Read the model definition and answer for the solid it produces. Units are mm, in the model's axes. A direction names the side the tool comes from. Give positions to 0.01 mm unless a question says otherwise; leave off trailing zeros. Loops run counter-clockwise (first coordinate to the right, second up) from the corner with the lowest first, then second, coordinate; pieces in that order, holes last. Notation, with made-up numbers: (36.5, 14) -> (49.5, 14) arc R7 cw to (49.5, 27) -> close; hole circle Ø5 at (59, 18). An arc over 180 degrees is marked (long way). Write each question's results on one line, items separated by ' | '. Start each with the question number.
Item 1: Which of the six approach directions +Z, -Z, +X, -X, +Y, -Y give full straight-line access (tool end or side, diameter ignored) to faces 1 (the flat face through (18.374, 8.986, 14.113)), 2 (the cylindrical face through (17.1, 1.97, 14.43)), 3 (the cylindrical face through (17.1, 2.29, 3.98)), 4 (the flat face through (22, 9, 1.5))?
Item 2: Each of these flat-tipped pins is pushed along its axis until it touches: P1, Ø2.5, axis at x = 16.65, y = 10, coming from the +Z side; P2, Ø2, axis at x = 24, y = 9.5, coming from the -Z side; P3, Ø1, axis at y = 3, z = 2.5, coming from the -X side. Where does it stop, or does it pass through?
Item 3: Section C-C on x = -4 is taken. Write down the section's boundary in (y, z), and give its area (3 significant figures).
Item 4: Find the intervals of material crossed by line 1 (X direction, y = 7.5, z = 7.5); line 2 (X direction, y = 1.3, z = 7.5); line 3 (X direction, y = 6.75, z = 11.5), in increasing order.
Item 5: Section A-A on x = 32.7 is taken. Write down the section's boundary in (y, z) (3 decimals).
Item 6: Section B-B on x = 17 is taken. State how many separate pieces and enclosed holes the cut face has, and give its area (3 significant figures).
Item 7: Determine the mould class of faces 5 (the flat face through (4, 4, 8)), 6 (the flat face through (23, 12, 14)), 7 (the cylindrical face through (46.727, 2.535, 7.142)) for opening direction Y: +Y half, -Y half, draft (parallel to the pull), parting line (faces both ways), or undercut.
```python
from build123d import *

# Parameters (mm, degrees)
SKETCH1_W                = 40
SKETCH1_H                = 13
SWITCHCASE_DEPTH         = 15
SKETCH2_W                = 13
SKETCH2_H                = 5.9
SWITCHCAVITY_DEPTH       = 45.654227124
SWITCHM2HOLES_DEPTH      = 44.338233697
SWITCHM2HOLES_DEPTH_BACK = 44.338233697
SKETCH3_R                = 1.05
SKETCH14_R               = 2
M2HEAD_DEPTH             = 1.5
M2NUTINSERTS_DEPTH       = 45.654227124
M2NUTINSERTS_DEPTH_BACK  = 1.75
SKETCH7_W                = 15
SKETCH7_H                = 13
WINGS_DEPTH              = 15
M5NUTS_DEPTH             = 4
SKETCH10_R               = 3.05
M6HOLE_DEPTH             = 59.472215624
WIRECHANNEL_DEPTH        = 58.473493891
WIRECHANNEL_DEPTH_BACK   = 58.473493891
SKETCH11_W               = 4.6
SKETCH11_H               = 4
CHANNELFILLET_R          = 2
M5HEAD_DEPTH             = 59.472215624
M5HEAD_DEPTH_BACK        = 8
SKETCH12_R               = 4.5
SKETCH13_R               = 2.75
M5THREAD_DEPTH           = 59.472215624
ENDFILLET_R              = 5


with BuildPart() as part:
    # Sketch1 → SwitchCase (new body)
    with BuildSketch(Plane.XY):
        with Locations((20, 6.5)):
            Rectangle(SKETCH1_W, SKETCH1_H)
    extrude(amount=SWITCHCASE_DEPTH)

    # Sketch2 → SwitchCavity (cut, through all)
    with BuildSketch(Plane(origin=(0, 13, 0), x_dir=(1, 0, 0), z_dir=(0, 1, 0))):
        with Locations((20, -7.5)):
            Rectangle(SKETCH2_W, SKETCH2_H)
    extrude(amount=-SWITCHCAVITY_DEPTH, mode=Mode.SUBTRACT)

    # Sketch3 → SwitchM2Holes (cut, two sides: drawn at the far end of the back side and taken through both)
    with BuildSketch(Plane.XY.offset(4.55).offset(-SWITCHM2HOLES_DEPTH_BACK)):
        with Locations((16.65, 10)):
            Circle(SKETCH3_R)
        with Locations((23.35, 10)):
            Circle(SKETCH3_R)
    extrude(amount=SWITCHM2HOLES_DEPTH + SWITCHM2HOLES_DEPTH_BACK, mode=Mode.SUBTRACT)

    # Sketch14 → M2Head (cut)
    with BuildSketch(Plane(origin=(0, 0, 0), x_dir=(-1, 0, 0), z_dir=(0, 0, -1))):
        with Locations((-23.35, 10)):
            Circle(SKETCH14_R)
        with Locations(Location((-16.65, 10, 0), (0, 0, 180))):
            Circle(SKETCH14_R)
    extrude(amount=-M2HEAD_DEPTH, mode=Mode.SUBTRACT)

    # Sketch5 → M2NutInserts (cut, two sides: drawn at the far end of the back side and taken through both)
    with BuildSketch(Plane.XY.offset(15).offset(-M2NUTINSERTS_DEPTH_BACK)):
        Polygon((18.959401077, 10), (17.804700538, 12), (15.495299462, 12), (14.340598923, 10), (15.495299462, 8), (17.804700538, 8), align=None)
        Polygon((25.659401077, 10), (24.504700538, 12), (22.195299462, 12), (21.040598923, 10), (22.195299462, 8), (24.504700538, 8), align=None)
    extrude(amount=M2NUTINSERTS_DEPTH + M2NUTINSERTS_DEPTH_BACK, mode=Mode.SUBTRACT)

    # Sketch7 → Wings (add)
    with BuildSketch(Plane.XY.offset(15)):
        with Locations((-7.5, 6.5)):
            Rectangle(SKETCH7_W, SKETCH7_H)
        with Locations((47.5, 6.5)):
            Rectangle(SKETCH7_W, SKETCH7_H)
    extrude(amount=-WINGS_DEPTH)

    # Sketch9 → M5Nuts (cut)
    with BuildSketch(Plane.XZ):
        Polygon((37.232199613, 7.5), (34.966099807, 11.425), (30.433900193, 11.425), (28.167800387, 7.5), (30.433900193, 3.575), (34.966099807, 3.575), align=None)
        Polygon((5.033900193, 3.575), (2.767800387, 7.5), (5.033900193, 11.425), (9.566099807, 11.425), (11.832199613, 7.5), (9.566099807, 3.575), align=None)
    extrude(amount=-M5NUTS_DEPTH, mode=Mode.SUBTRACT)

    # Sketch10 → M6Hole (cut, through all)
    with BuildSketch(Plane.XZ):
        with Locations(Location((7.3, 7.5, 0), (0, 0, 270))):
            Circle(SKETCH10_R)
        with Locations(Location((32.7, 7.5, 0), (0, 0, 270))):
            Circle(SKETCH10_R)
    extrude(amount=-M6HOLE_DEPTH, mode=Mode.SUBTRACT)

    # Sketch11 → WireChannel (cut, two sides: drawn at the far end of the back side and taken through both)
    with BuildSketch(Plane.XY.offset(4.55).offset(-WIRECHANNEL_DEPTH_BACK)):
        with Locations((20, 2)):
            Rectangle(SKETCH11_W, SKETCH11_H)
    extrude(amount=WIRECHANNEL_DEPTH + WIRECHANNEL_DEPTH_BACK, mode=Mode.SUBTRACT)

    # ChannelFillet
    channelfillet_edges = [part.edges().sort_by_distance(p)[0] for p in [
        (20, 4, 10.45),
        (17.7, 2, 10.45),
        (22.3, 2, 10.45),
        (22.3, 2, 4.55),
        (22.3, 2, 0),
        (17.7, 2, 4.55),
        (17.7, 2, 0),
        (20, 4, 4.55),
        (22.3, 2, 15),
        (17.7, 2, 15),
    ]]
    fillet(channelfillet_edges, radius=CHANNELFILLET_R)

    # Sketch12 → M5Head (cut, two sides: drawn at the far end of the back side and taken through both)
    with BuildSketch(Plane(origin=(0, 13, 0), x_dir=(1, 0, 0), z_dir=(0, 1, 0)).offset(-M5HEAD_DEPTH_BACK)):
        with Locations(Location((44, -7.5, 0), (0, 0, 90))):
            Circle(SKETCH12_R)
        with Locations(Location((-4, -7.5, 0), (0, 0, 90))):
            Circle(SKETCH12_R)
    extrude(amount=M5HEAD_DEPTH + M5HEAD_DEPTH_BACK, mode=Mode.SUBTRACT)

    # Sketch13 → M5Thread (cut, through all)
    with BuildSketch(Plane(origin=(0, 13, 0), x_dir=(1, 0, 0), z_dir=(0, 1, 0))):
        with Locations(Location((44, -7.5, 0), (0, 0, 270))):
            Circle(SKETCH13_R)
        with Locations(Location((-4, -7.5, 0), (0, 0, 90))):
            Circle(SKETCH13_R)
    extrude(amount=-M5THREAD_DEPTH, mode=Mode.SUBTRACT)

    # EndFillet
    endfillet_edges = [part.edges().sort_by_distance(p)[0] for p in [
        (-15, 6.5, 15),
        (-15, 6.5, 0),
        (55, 6.5, 15),
        (55, 6.5, 0),
    ]]
    fillet(endfillet_edges, radius=ENDFILLET_R)


solid = part.part
```
Findings:
1) face 1: +Z | face 2: +Z, -Y | face 3: -Y | face 4: -Z
2) P1: z = 13.25 | P2: z = 1.5 | P3: x = -14.58
3) outline: (0, 0) -> (13, 0) -> (13, 3) -> (5, 3) -> (5, 4.75) -> (0, 4.75) -> close; (0, 10.25) -> (5, 10.25) -> (5, 12) -> (13, 12) -> (13, 15) -> (0, 15) -> close | area: 95.5 mm2
4) line 1: -15 to -8.5, 0.5 to 4.25, 10.35 to 13.5, 26.5 to 29.65, 35.75 to 39.5, 48.5 to 55 | line 2: -15 to -6.75, -1.25 to 2.77, 11.83 to 13.5, 26.5 to 28.17, 37.23 to 41.25, 46.75 to 55 | line 3: -14.77 to -6.06, -1.94 to 41.94, 46.06 to 54.77
5) outline: (0, 0) -> (13, 0) -> (13, 4.45) -> (4, 4.45) -> (4, 3.575) -> (0, 3.575) -> close; (0, 11.425) -> (4, 11.425) -> (4, 10.55) -> (13, 10.55) -> (13, 15) -> (0, 15) -> close
6) separate pieces: 4 | enclosed holes: 0 | area: 85.1 mm2
7) face 5: -Y half | face 6: undercut | face 7: draft
